Verification items for the finished model (mm, model axes). Face numbers are marked on the shaded views. A direction names the side the tool comes from. Give positions to 0.01 mm unless a question says otherwise; leave off trailing zeros. Loops run counter-clockwise (first coordinate to the right, second up) from the corner with the lowest first, then second, coordinate; pieces in that order, holes last. Notation, with made-up numbers: M 70.25,42.5 L 83.25,42.5 A19 ccw 83.25,47.5 Z; hole C 62,-1 d10. An arc over 180 degrees is marked long. Answer in a Markdown table with one row per item.
```python
from build123d import *

# Parameters (mm, degrees)
F1_DEPTH = 228.6
F3_DEPTH = 6.35
F4_R     = 10.31875
F5_DEPTH = 25.4


with BuildPart() as f1:
    # F0 (on Right) → F1 (new body, symmetric)
    with BuildSketch(Plane.YZ):
        Polygon((101.6, 142.875), (101.6, 152.4), (-101.6, 152.4), (-101.6, -152.4), (-92.075, -152.4), (-92.075, 142.875), align=None)
    extrude(amount=F1_DEPTH, both=True)

    # F2 (on Right) → F3 (join, symmetric)
    with BuildSketch(Plane.YZ):
        Polygon((-92.075, -152.4), (101.6, 142.875), (-92.075, 142.875), align=None)
    extrude(amount=F3_DEPTH, both=True)

    # F4 (on face) → F5 (cut)
    with BuildSketch(Plane(origin=(0, -92.075, 0), x_dir=(-1, 0, 0), z_dir=(0, 1, 0))):
        with Locations((-162.71875, 0)):
            Circle(F4_R)
        with Locations((162.71875, 0)):
            Circle(F4_R)
    extrude(amount=-F5_DEPTH, mode=Mode.SUBTRACT)


solid = f1.part
```
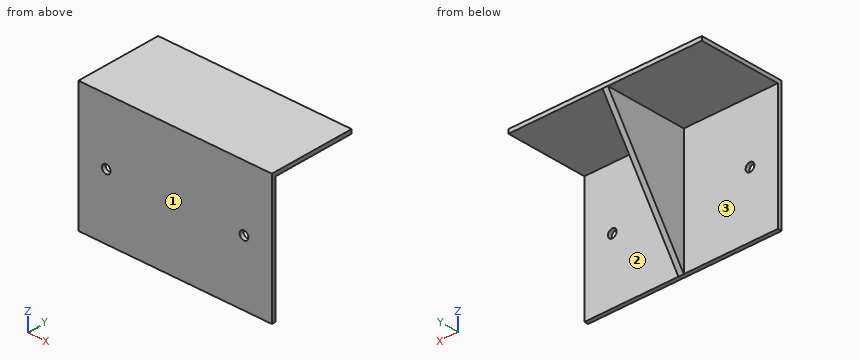
Item 1: Go/stop test with flat-tipped pins: pin 1 (1.5 mm diameter, centred on x = -180.5, z = 10.5, fed in from +Y) (3 decimals); pin 2 (12 mm diameter, centred on x = -74.5, y = -64.5, fed in from -Z) (3 decimals); pin 3 (1.5 mm diameter, centred on y = 55.5, z = 111.5, fed in from +X); pin 4 (12.5 mm diameter, centred on x = -162.72, z = 0, fed in from +Y). Record where each tip stops, or that it passes through.
Reported:
| item | result |
|---|---|
| pin 1 | stops at y = -92.075 |
| pin 2 | stops at z = 142.875 |
| pin 3 | stops at x = 6.35 |
| pin 4 | passes through |
Item 2: Sectioned sample at C-C (y = 53). Record the cut outline in (x, z) (3 decimals), and give its area (3 significant figures).
Reported:
| item | result |
|---|---|
| outline | M -228.6,142.875 L -6.35,142.875 L -6.35,68.78 L 6.35,68.78 L 6.35,142.875 L 228.6,142.875 L 228.6,152.4 L -228.6,152.4 Z |
| area | 5,300 mm^2 |
Item 3: Sectioned sample at A-A (z = 0). State how many separate pieces and enclosed holes the cut face has, and give its area (3 significant figures).
Reported:
| item | result |
|---|---|
| separate pieces | 3 |
| enclosed holes | 0 |
| area | 5,230 mm^2 |
Item 4: Tool access check on the marked faces 1, 2 and 3. Record the directions out of +Z, -Z, +X, -X, +Y, -Y that give a thin tool (end or side, any length) a straight path to the whole face; none if there is none.
Reported:
| item | result |
|---|---|
| face 1 | +Z, -Z, +X, -X, -Y |
| face 2 | -Z, +X, +Y |
| face 3 | -Z, -X, +Y |
Item 5: Scan lines: L1, parallel to Y at x = -193, z = -113.5 (3 decimals); L2, parallel to X at y = -63.5, z = 39; L3, parallel to Z at x = -46.5, y = -31 (3 decimals). Record each from-to range of solid material in increasing order. Write a range as [from, to].
Reported:
| item | result |
|---|---|
| L1 | y = [-101.6, -92.075] |
| L2 | x = [-6.35, 6.35] |
| L3 | z = [142.875, 152.4] |
Item 6: Sectioned sample at D-D (z = -51.5). Record the cut outline in (x, y) (3 decimals), and give its area (3 significant figures).
Reported:
| item | result |
|---|---|
| outline | M -228.6,-101.6 L 228.6,-101.6 L 228.6,-92.075 L 6.35,-92.075 L 6.35,-25.893 L -6.35,-25.893 L -6.35,-92.075 L -228.6,-92.075 Z |
| area | 5,200 mm^2 |
Item 7: Sectioned sample at B-B (x = 192.5). Record the cut outline in (y, z) (3 decimals), and give its area (3 significant figures).
Reported:
| item | result |
|---|---|
| outline | M -101.6,-152.4 L -92.075,-152.4 L -92.075,142.875 L 101.6,142.875 L 101.6,152.4 L -101.6,152.4 Z |
| area | 4,750 mm^2 |
